Build history of the part. All positions in model axes, mm. A direction names the side the tool comes from. Coordinates: 2 decimals unless noted, no trailing zeros. Loops run counter-clockwise (first coordinate to the right, second up) from the corner with the lowest first, then second, coordinate; pieces in that order, holes last. Notation, with made-up numbers: (10, 16.25) - (69, 16.25) arc R10 cw to (69, 22.25) - close; hole circle Ø4 at (74, 60.5). An arc over 180 degrees is marked (long way). One line per item, written item: value.
```python
from build123d import *

# Parameters (mm, degrees)
SKETCH1_R           = 2
SKETCH1_R_2         = 3.05
BOSS_EXTRUDE1_DEPTH = 20
SKETCH2_R           = 2.2
CUT_EXTRUDE1_DEPTH  = 27.508
SKETCH2_3_R         = 3.7
SKETCH2_3_R_2       = 2.2
CUT_EXTRUDE2_DEPTH  = 6.435712
BOSS_EXTRUDE2_START = 6.3
SKETCH1_2_R         = 3.05
BOSS_EXTRUDE2_DEPTH = 13.7
FILLET1_R           = 2


with BuildPart() as part:
    # Sketch1 → Boss-Extrude1 (new body)
    with BuildSketch(Plane.XY):
        Polygon((-15.2, -92.57905153), (-50.600589502, -92.57905153), (-50.600589502, -84.143339933), (-43.100589502, -84.143339933), (-43.100589502, -82.343339933), (-38.100589502, -82.343339933), (-38.100589502, -84.143339933), (-30.600589502, -84.143339933), (-30.600589502, -69.503339933), (-15.2, -69.503339933), align=None)
        with Locations((-25.300294751, -84.31585339)):
            Circle(SKETCH1_R, mode=Mode.SUBTRACT)
        with Locations((-19.300294751, -84.31585339)):
            Circle(SKETCH1_R, mode=Mode.SUBTRACT)
        with Locations((-22.300294751, -77.31585339)):
            Circle(SKETCH1_R_2, mode=Mode.SUBTRACT)
    extrude(amount=BOSS_EXTRUDE1_DEPTH)

    # Sketch2 → Cut-Extrude1 (cut)
    with BuildSketch(Plane.XZ.offset(92.57905153)):
        with Locations((-40.600589502, 10)):
            Circle(SKETCH2_R)
    extrude(amount=-CUT_EXTRUDE1_DEPTH, mode=Mode.SUBTRACT)

    # Sketch2<3> → Cut-Extrude2 (cut)
    with BuildSketch(Plane.XZ.offset(92.57905153)):
        with Locations((-40.600589502, 10)):
            Circle(SKETCH2_3_R)
        with Locations((-40.600589502, 10)):
            Circle(SKETCH2_3_R_2, mode=Mode.SUBTRACT)
    extrude(amount=-CUT_EXTRUDE2_DEPTH, mode=Mode.SUBTRACT)

    # Sketch1<2> → Boss-Extrude2 (add)
    with BuildSketch(Plane.XY.offset(BOSS_EXTRUDE2_START)):
        with Locations((-22.300294751, -77.31585339)):
            Circle(SKETCH1_2_R)
    extrude(amount=BOSS_EXTRUDE2_DEPTH)

    # Fillet1
    fillet1_edges = [part.edges().sort_by_distance(p)[0] for p in [
        (-32.900294751, -92.57905153, 0),
        (-50.600589502, -88.361195731, 0),
        (-30.600589502, -76.823339933, 20),
        (-30.600589502, -76.823339933, 0),
        (-22.900294751, -69.503339933, 0),
        (-15.2, -81.041195731, 0),
        (-15.2, -92.57905153, 10),
        (-50.600589502, -92.57905153, 10),
        (-50.600589502, -84.143339933, 10),
        (-30.600589502, -69.503339933, 10),
        (-15.2, -69.503339933, 10),
        (-50.600589502, -88.361195731, 20),
        (-32.900294751, -92.57905153, 20),
        (-15.2, -81.041195731, 20),
        (-22.900294751, -69.503339933, 20),
    ]]
    fillet(fillet1_edges, radius=FILLET1_R)


solid = part.part
```
Item 1: Cut at B-B, the plane z = 10. Write the cut outline in (x, y), then the cut area to 3 significant figures.
Check result:
outline: (-50.6, -90.58) arc R2 ccw to (-48.6, -92.58) - (-44.3, -92.58) - (-44.3, -86.14) - (-42.8, -86.14) - (-42.8, -82.34) - (-43.1, -82.34) - (-43.1, -84.14) - (-48.6, -84.14) arc R2 ccw to (-50.6, -86.14) - close; (-38.4, -86.14) - (-36.9, -86.14) - (-36.9, -92.58) - (-17.2, -92.58) arc R2 ccw to (-15.2, -90.58) - (-15.2, -71.5) arc R2 ccw to (-17.2, -69.5) - (-28.6, -69.5) arc R2 ccw to (-30.6, -71.5) - (-30.6, -84.14) - (-38.1, -84.14) - (-38.1, -82.34) - (-38.4, -82.34) - close; hole circle Ø4 at (-25.3, -84.32); hole circle Ø4 at (-19.3, -84.32)
area: 439 mm^2
Item 2: Probe probe 1 along X at (y, z) = (-83, 9.75); probe 2 along Y at (x, z) = (-25, 6.25); probe 3 along X at (y, z) = (-73.75, 12). List the from-to ranges inside material, lowest first. Write a range as from..to.
Check result:
probe 1: x = -43.1..-42.79, -38.41..-38.1, -30.6..-26.81, -23.79..-20.81, -17.79..-15.2
probe 2: y = -92.58..-86.29, -82.34..-78.74, -75.9..-69.5
probe 3: x = -30.6..-15.2
Item 3: Tool access for faces 1 (the face through (-37.07, -89.41, 11.11)), 2 (the face through (-38.101, -83, 10)), 3 (the face through (-40.6, -82.343, 7.6)): list every direction of +Z, -Z, +X, -X, +Y, -Y with a clear straight run to the whole face (end or side of a thin tool).
Check result:
face 1: -Y
face 2: +Z, -Z, +Y
face 3: +Z, -Z, -X, +Y
Item 4: Cut at D-D, the plane z = 14.75. Write the cut outline in (x, y), then the cut area to 3 significant figures.
Check result:
outline: (-50.6, -90.58) arc R2 ccw to (-48.6, -92.58) - (-17.2, -92.58) arc R2 ccw to (-15.2, -90.58) - (-15.2, -71.5) arc R2 ccw to (-17.2, -69.5) - (-28.6, -69.5) arc R2 ccw to (-30.6, -71.5) - (-30.6, -84.14) - (-38.1, -84.14) - (-38.1, -82.34) - (-43.1, -82.34) - (-43.1, -84.14) - (-48.6, -84.14) arc R2 ccw to (-50.6, -86.14) - close; hole circle Ø4 at (-25.3, -84.32); hole circle Ø4 at (-19.3, -84.32)
area: 504 mm^2
Item 5: Cut at A-A, the plane y = -83. Write the cut outline in (x, z).
Check result:
outline: (-43.1, 0) - (-38.1, 0) - (-38.1, 20) - (-43.1, 20) - close; (-30.6, 2) arc R2 ccw to (-28.6, 0) - (-26.81, 0) - (-26.81, 20) - (-28.6, 20) arc R2 ccw to (-30.6, 18) - close; (-23.79, 0) - (-20.81, 0) - (-20.81, 20) - (-23.79, 20) - close; (-17.79, 0) - (-17.2, 0) arc R2 ccw to (-15.2, 2) - (-15.2, 18) arc R2 ccw to (-17.2, 20) - (-17.79, 20) - close; hole circle Ø4.4 at (-40.6, 10)
Item 6: Cut at C-C, the plane x = -32.5. Write the cut outline in (y, z).
Check result:
outline: (-92.58, 2) arc R2 ccw to (-90.58, 0) - (-84.14, 0) - (-84.14, 20) - (-90.58, 20) arc R2 ccw to (-92.58, 18) - close
Item 7: Drop flat-ended pins along their axis: P1, Ø4.5, axis at x = -40.6, z = 10, coming from the +Y side; P2, Ø3.5, axis at x = -40.5, z = 8.5, coming from the -Y side; P3, Ø10, axis at y = -79, z = 5, coming from the -X side. Give the stop position or say it passes through.
Check result:
P1: stops at y = -82.34
P2: stops at y = -86.14
P3: stops at x = -43.1
Item 8: Pull direction Z, two halves, no side cores. Call faces 4 (the face through (-30.03, -77.73, 19.4)), 5 (the face through (-15.2, -81, 10)), 6 (the face through (-39, -86.143, 8)): released by +Z, released by -Z, zero draft, split by the parting line, or undercut.
Check result:
face 4: released by +Z
face 5: zero draft
face 6: undercut
